Can you work these out from the model? Positions are in its coordinate system, mm. A direction names the side the tool comes from. Give positions to 0.01 mm unless a question says otherwise; leave off trailing zeros. Write each loop counter-clockwise with the first axis right and the second up, starting at its lowest first coordinate (ties: lowest second). Pieces come first, ordered by that corner, then holes.
from build123d import *

# Parameters (mm, degrees)
BOSS_EXTRUDE1_DEPTH = 12
CUT_EXTRUDE1_DEPTH  = 13


with BuildPart() as part:
    # Sketch1 → Boss-Extrude1 (new body)
    with BuildSketch(Plane(origin=(0, 0, 0), x_dir=(1, 0, 0), z_dir=(0, 1, 0))):
        with BuildLine():
            Line((-1.209935044, 20.498962969), (-1.209935044, 14.951122272))
            ThreePointArc((-1.209935044, 14.951122272), (-4.085137635, 14.433005595), (-6.805373075, 13.367381842))
            Line((-6.805373075, 13.367381842), (-9.565265163, 18.147655161))
            ThreePointArc((-9.565265163, 18.147655161), (-11.431290566, 19.379705968), (-11.29731597, 17.147655161))
            Line((-11.29731597, 17.147655161), (-8.523395621, 12.34308418))
            ThreePointArc((-8.523395621, 12.34308418), (-10.754335768, 10.45678068), (-12.577316886, 8.17380572))
            Line((-12.577316886, 8.17380572), (-17.357590205, 10.933697807))
            ThreePointArc((-17.357590205, 10.933697807), (-19.589641013, 11.067672403), (-18.357590205, 9.201646999))
            Line((-18.357590205, 9.201646999), (-13.553019225, 6.427726651))
            ThreePointArc((-13.553019225, 6.427726651), (-14.541918316, 3.678669827), (-14.979178795, 0.790064956))
            Line((-14.979178795, 0.790064956), (-20.498962969, 0.790064956))
            ThreePointArc((-20.498962969, 0.790064956), (-22.498962969, -0.209935044), (-20.498962969, -1.209935044))
            Line((-20.498962969, -1.209935044), (-14.951122272, -1.209935044))
            ThreePointArc((-14.951122272, -1.209935044), (-14.433005595, -4.085137635), (-13.367381842, -6.805373075))
            Line((-13.367381842, -6.805373075), (-18.147655161, -9.565265163))
            ThreePointArc((-18.147655161, -9.565265163), (-19.379705968, -11.431290566), (-17.147655161, -11.29731597))
            Line((-17.147655161, -11.29731597), (-12.34308418, -8.523395621))
            ThreePointArc((-12.34308418, -8.523395621), (-10.45678068, -10.754335768), (-8.17380572, -12.577316886))
            Line((-8.17380572, -12.577316886), (-10.933697807, -17.357590205))
            ThreePointArc((-10.933697807, -17.357590205), (-11.067672403, -19.589641013), (-9.201646999, -18.357590205))
            Line((-9.201646999, -18.357590205), (-6.427726651, -13.553019225))
            ThreePointArc((-6.427726651, -13.553019225), (-3.678669827, -14.541918316), (-0.790064956, -14.979178795))
            Line((-0.790064956, -14.979178795), (-0.790064956, -20.498962969))
            ThreePointArc((-0.790064956, -20.498962969), (0.209935044, -22.498962969), (1.209935044, -20.498962969))
            Line((1.209935044, -20.498962969), (1.209935044, -14.951122272))
            ThreePointArc((1.209935044, -14.951122272), (4.085137635, -14.433005595), (6.805373075, -13.367381842))
            Line((6.805373075, -13.367381842), (9.565265163, -18.147655161))
            ThreePointArc((9.565265163, -18.147655161), (11.431290566, -19.379705968), (11.29731597, -17.147655161))
            Line((11.29731597, -17.147655161), (8.523395621, -12.34308418))
            ThreePointArc((8.523395621, -12.34308418), (10.754335768, -10.45678068), (12.577316886, -8.17380572))
            Line((12.577316886, -8.17380572), (17.357590205, -10.933697807))
            ThreePointArc((17.357590205, -10.933697807), (19.589641013, -11.067672403), (18.357590205, -9.201646999))
            Line((18.357590205, -9.201646999), (13.553019225, -6.427726651))
            ThreePointArc((13.553019225, -6.427726651), (14.541918316, -3.678669827), (14.979178795, -0.790064956))
            Line((14.979178795, -0.790064956), (20.498962969, -0.790064956))
            ThreePointArc((20.498962969, -0.790064956), (22.498962969, 0.209935044), (20.498962969, 1.209935044))
            Line((20.498962969, 1.209935044), (14.951122272, 1.209935044))
            ThreePointArc((14.951122272, 1.209935044), (14.433005595, 4.085137635), (13.367381842, 6.805373075))
            Line((13.367381842, 6.805373075), (18.147655161, 9.565265163))
            ThreePointArc((18.147655161, 9.565265163), (19.379705968, 11.431290566), (17.147655161, 11.29731597))
            Line((17.147655161, 11.29731597), (12.34308418, 8.523395621))
            ThreePointArc((12.34308418, 8.523395621), (10.45678068, 10.754335768), (8.17380572, 12.577316886))
            Line((8.17380572, 12.577316886), (10.933697807, 17.357590205))
            ThreePointArc((10.933697807, 17.357590205), (11.067672403, 19.589641013), (9.201646999, 18.357590205))
            Line((9.201646999, 18.357590205), (6.427726651, 13.553019225))
            ThreePointArc((6.427726651, 13.553019225), (3.678669827, 14.541918316), (0.790064956, 14.979178795))
            Line((0.790064956, 14.979178795), (0.790064956, 20.498962969))
            ThreePointArc((0.790064956, 20.498962969), (-0.209935044, 22.498962969), (-1.209935044, 20.498962969))
        make_face()
    extrude(amount=BOSS_EXTRUDE1_DEPTH)

    # Sketch2 → Cut-Extrude1 (cut, through all)
    with BuildSketch(Plane(origin=(0, 12, 0), x_dir=(1, 0, 0), z_dir=(0, 1, 0))):
        with BuildLine():
            Line((-2.236067977, 2), (2.236067977, 2))
            ThreePointArc((2.236067977, 2), (0, -3), (-2.236067977, 2))
        make_face()
    extrude(amount=-CUT_EXTRUDE1_DEPTH, mode=Mode.SUBTRACT)


solid = part.part
(1) Imagine slicing it at C-C, the plane x = -4.5. Write out the boundary of the cut face in (y, z), plus the area to 3 significant figures.
Returned:
outline: (0, -14.31) - (12, -14.31) - (12, 14.31) - (0, 14.31) - close
area: 343 mm2
(2) Imagine slicing it at A-A, the plane x = 0. Write out the boundary of the cut face in (y, z).
Returned:
outline: (0, -22.48) - (12, -22.48) - (12, -2) - (0, -2) - close; (0, 3) - (12, 3) - (12, 22.48) - (0, 22.48) - close
(3) For faces 5 (the face through (-0.79, 6, 18)), 6 (the face through (15.989, 5.916, 7.834)), 7 (the face through (-15.724, 5.916, 8.166)), which set-ups out of +Z, -Z, +X, -X, +Y, -Y let a thin tool reach every point of the face, with its end or its side?
Returned:
face 5: +Y, -Y
face 6: +X, +Y, -Y
face 7: -X, +Y, -Y
(4) Will these pins go through, and if not, where does the flat tip stop? P1, Ø6, axis at y = 4.5, z = 17.5, coming from the +X side; P2, Ø4.5, axis at y = 4, z = -17, coming from the -X side; P3, Ø6, axis at x = 7, y = 7, coming from the -Z side.
Returned:
P1: stops at x = 12.06
P2: stops at x = -12.06
P3: stops at z = -19.68
(5) If we mould it in two halves opening along X, with no side actions, what happens to faces 1 (the face through (-9.53, 5.92, 14.93)), 2 (the face through (3.72, 5.92, -14.53)), 3 (the face through (-0.2, 5.9, -22.5)), 4 (the face through (-3.72, 5.92, 14.53))? For each: +X half, -X half, draft (parallel to the pull), parting line (faces both ways), or undercut.
Returned:
face 1: -X half
face 2: undercut
face 3: parting line
face 4: undercut
(6) If I drill on L1, parallel to X at y = 3.75, z = -17; L2, parallel to Z at x = 16.5, y = 7.5; L3, parallel to X at y = 2, z = 16, over which ranges is the centre line in solid material (lowest first)?
Returned:
L1: x = -11.21 to -8.9, -1.21 to 0.79, 8.42 to 10.73
L2: z = -10.92 to -8.61, -1.21 to 0.79, 8.13 to 10.44
L3: x = -10.15 to -7.84, -0.79 to 1.21, 8.33 to 10.63
(7) Imagine slicing it at B-B, the plane z = 0. Write out the boundary of the cut face in (x, y), plus the area to 3 significant figures.
Returned:
outline: (-22.48, 0) - (-3, 0) - (-3, 12) - (-22.48, 12) - close; (3, 0) - (22.48, 0) - (22.48, 12) - (3, 12) - close
area: 468 mm2
